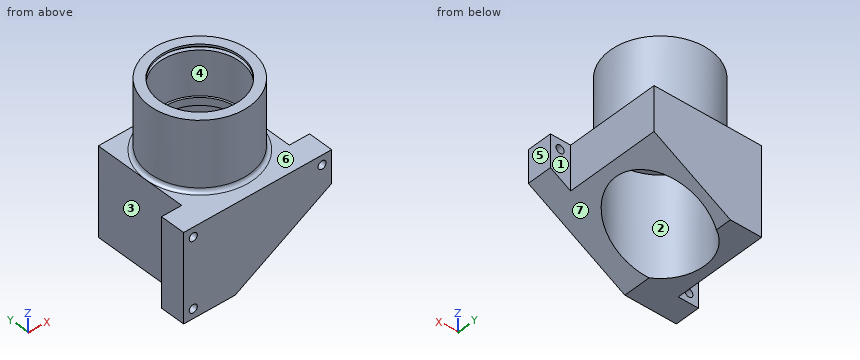
```python
from build123d import *

# Parameters (mm, degrees)
SKETCH_1_W          = 56
SKETCH_1_H          = 62
EXTRUDE_1_DEPTH     = 82
SKETCH_4_W          = 56
SKETCH_4_H          = 62
SKETCH_4_R          = 26
CUT_EXTRUDE_1_DEPTH = 36
SKETCH_15_W         = 23
SKETCH_15_H         = 1.9
FILLET_1_R          = 2
SKETCH_19_W         = 10.5
SKETCH_19_H         = 46
EXTRUDE_2_DEPTH     = 13
CUT_EXTRUDE_2_DEPTH = 110.773630713
HOLE_WIZARD_M5_1_D  = 4.2


with BuildPart() as part:
    # 草图1 → 凸台-拉伸1 (new body)
    with BuildSketch(Plane.XY):
        with Locations((0, -3)):
            Rectangle(SKETCH_1_W, SKETCH_1_H)
    extrude(amount=EXTRUDE_1_DEPTH)

    # 草图3 → 切除-旋转2 (revolve, cut)
    with BuildSketch(Plane(origin=(0, 0, 0), x_dir=(0, 0, -1), z_dir=(1, 0, 0)), mode=Mode.PRIVATE) as cut_revolve_2_sk:
        Polygon((-82, 0), (0, 0), (0, 23), (-52, 23), (-52, 20), (-56, 20), (-56, 21), (-82, 21), align=None)
    revolve(cut_revolve_2_sk.sketch.rotate(Axis((0, 0, -5.719261836), (0, 0, 1)), 90), axis=Axis((0, 0, -5.719261836), (0, 0, 1)), mode=Mode.SUBTRACT)

    # 草图4 → 切除-拉伸1 (cut)
    with BuildSketch(Plane.XY.offset(82)):
        with Locations((0, -3)):
            Rectangle(SKETCH_4_W, SKETCH_4_H)
        Circle(SKETCH_4_R, mode=Mode.SUBTRACT)
    extrude(amount=-CUT_EXTRUDE_1_DEPTH, mode=Mode.SUBTRACT)

    # 草图15 → 切除-旋转3 (revolve, cut)
    with BuildSketch(Plane(origin=(0, 0, 0), x_dir=(1, 0, 0), z_dir=(0, 1, 0))):
        with Locations((-11.5, -79.95)):
            Rectangle(SKETCH_15_W, SKETCH_15_H)
    revolve(axis=Axis((0, 0, 0), (0, 0, 1)), mode=Mode.SUBTRACT)

    # 圆角1
    fillet_1_edges = [part.edges().sort_by_distance(p)[0] for p in [
        (-26, 0, 46),
    ]]
    fillet(fillet_1_edges, radius=FILLET_1_R - 0.0001)  # a hair under: the kernel refuses the full size

    # 草图19 → 凸台-拉伸2 (add)
    with BuildSketch(Plane.XZ.offset(34)):
        with Locations((33.25, 23)):
            Rectangle(SKETCH_19_W, SKETCH_19_H)
        with Locations((-33.25, 23)):
            Rectangle(SKETCH_19_W, SKETCH_19_H)
    extrude(amount=-EXTRUDE_2_DEPTH)

    # 草图25 → 切除-拉伸2 (cut, through all)
    with BuildSketch(Plane.XZ.offset(34)):
        Polygon((213.716550827, 130.161322786), (38.5, 29), (-11.729473419, 0), (-186.946024246, -101.161322786), (15.376621326, -451.59442444), (416.039196399, -220.271778867), align=None)
    extrude(amount=-CUT_EXTRUDE_2_DEPTH, mode=Mode.SUBTRACT)

    # M5 螺纹孔1 (through all)
    with Locations(Plane(origin=(0, -34, 0), x_dir=(-1, 0, 0), z_dir=(0, -1, 0))):
        with Locations((33.5, -5), (-33.5, -41), (33.5, -41)):
            Hole(HOLE_WIZARD_M5_1_D / 2)


solid = part.part
```
Work out the finished part from the listing and answer in its coordinate system (mm). Face numbers are marked on the shaded views. A direction names the side the tool comes from. Give positions to 0.01 mm unless a question says otherwise; leave off trailing zeros. Loops run counter-clockwise (first coordinate to the right, second up) from the corner with the lowest first, then second, coordinate; pieces in that order, holes last. Notation, with made-up numbers: (9.5, 39.25) - (59.5, 39.25) arc R16 ccw to (59.5, 61.25) - close; hole circle Ø7 at (61, -38.75). An arc over 180 degrees is marked (long way). Use CSV: the item, a comma, the result in double quotes. Start each with the question number.
(1) Find section B-B, the plane x = -33.5. Determine the outline of the cut face in (y, z).
(2) Determine the mould class of the marked faces 5, 6 and 7 for opening direction Z: released by +Z, released by -Z, zero draft, split by the parting line, or undercut.
(3) Each of these flat-tipped pins is pushed along its axis until it touches: pin 1 (5.5 mm diameter, centred on x = -33.5, z = 41, fed in from +Y); pin 2 (6 mm diameter, centred on y = -18.5, z = 59.5, fed in from +X); pin 3 (1 mm diameter, centred on x = 5, z = 9, fed in from +Y); pin 4 (8 mm diameter, centred on x = -28, z = 65.5, fed in from +Y). Where does it stop, or does it pass through?
(4) A tool of negligible diameter and unlimited length cuts with its end or side. For the marked faces 1, 2, 3 and 4, from which of +Z, -Z, +X, -X, +Y, -Y can it reach the whole face along a straight path? Write none if from no direction.
(5) Find the intervals of material crossed by L1, parallel to X at y = -26, z = 41; L2, parallel to Y at x = 0, z = 54.25; L3, parallel to Z at x = -20, y = -19.5, in increasing order.
(6) Find section D-D, the plane z = 70.5. Determine the outline of the cut face in (x, y), plus the area to 3 significant figures.
(7) Find section A-A, the plane z = 41. Determine the outline of the cut face in (x, y).
Results found:
1,outline,"(-34, 0) - (-21, 0) - (-21, 2.9) - (-34, 2.9) - close; (-34, 7.1) - (-21, 7.1) - (-21, 38.9) - (-34, 38.9) - close; (-34, 43.1) - (-21, 43.1) - (-21, 46) - (-34, 46) - close"
2,face 5,"zero draft"
2,face 6,"released by +Z"
2,face 7,"released by -Z"
3,pin 1,"y = -21"
3,pin 2,"x = 20.87"
3,pin 3,"through"
3,pin 4,"y = 10"
4,face 1,"+Z, -Z, +X, +Y"
4,face 2,"-Z"
4,face 3,"+Z, -Z, -X, +Y"
4,face 4,"+Z"
5,L1,"-38.5 to -35.6, -31.4 to 31.4, 35.6 to 38.5"
5,L2,"-26 to -20, 20 to 26"
5,L3,"0 to 46"
6,outline,"circle Ø52 at (0, 0); hole circle Ø42 at (0, 0)"
6,area,"738 mm^2"
7,outline,"(-38.5, -34) - (-35.6, -34) - (-35.6, -21) - (-38.5, -21) - close; (-31.4, -34) - (31.4, -34) - (31.4, -21) - (28, -21) - (28, 28) - (-28, 28) - (-28, -21) - (-31.4, -21) - close; (35.6, -34) - (38.5, -34) - (38.5, -21) - (35.6, -21) - close; hole circle Ø46 at (0, 0)"
